Autodesk Inventor part; units mm, degrees
ref_plane "YZ Plane" through (0, 0, 0) normal (1, 0, 0) x (0, 1, 0)
ref_plane "XZ Plane" through (0, 0, 0) normal (0, 1, 0) x (-1, 0, 0)
ref_plane "XY Plane" through (0, 0, 0) normal (0, 0, 1) x (1, 0, 0)
sketch "Sketch1" plane through (0, 0, 0) normal (0, 0, 1) x (1, 0, 0)
  line L0 (-12.4142, 25.4) -> (12.4142, 25.4)
  line L1 (12.4142, 25.4) -> (12.4142, -25.4)
  line L2 (12.4142, -25.4) -> (-12.4142, -25.4)
  line L3 (-12.4142, -25.4) -> (-12.4142, 25.4)
  circle A0 centre (-9.2393, 22.225) radius 2.1844
  circle A1 centre (-9.2393, -22.225) radius 2.1844
  circle A2 centre (9.2393, -22.225) radius 2.1844
  circle A3 centre (9.2393, 22.225) radius 2.1844
  point P0 (0, 0)
  point P1 (-12.4143, 0)
  point P2 (0, 25.4)
  dimension "d0" = 24.8285
  dimension "d1" = 50.8
  dimension "d2" = 4.3688
  dimension "d3" = 47.625
  dimension "d4" = 3.175
  dimension "d5" = 4.3688
  dimension "d6" = 4.3688
  dimension "d7" = 4.3688
  dimension "d8" = 3.175
  dimension "d9" = 3.175
extrude "Extrusion1" add sketch "Sketch1" against normal blind 9.398
properties part number "Ch7(5) Part 9 Cover Plate"
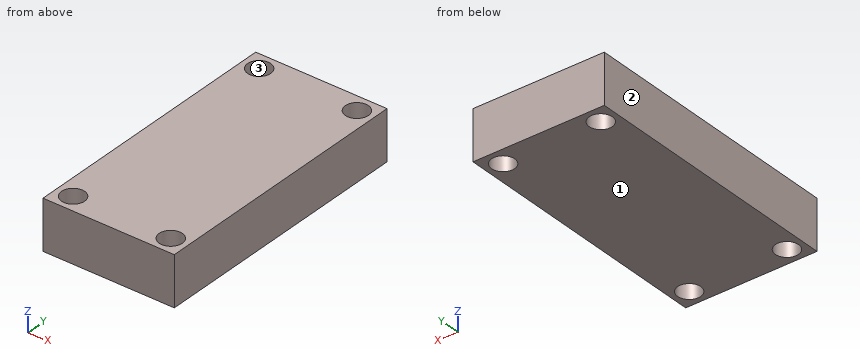
Geometry: final body of the model. Coordinates: model frame, mm. Face numbers are marked on the shaded views. Give positions to 0.01 mm unless a question says otherwise; leave off trailing zeros. Write each loop counter-clockwise with the first axis right and the second up, starting at its lowest first coordinate (ties: lowest second). Pieces come first, ordered by that corner, then holes. Notation, with made-up numbers: M -34,-6 L 23,-6 A5 cw 23,2 Z; hole C -20,33 d4. An arc over 180 degrees is marked long. Answer in a Markdown table with one row per item. Add a question column.
(1) Ray query, line 1 (Y direction, x = -9.25, z = -2); line 2 (Y direction, x = 11, z = -2.5); line 3 (X direction, y = 23.5, z = -8). Return the intervals inside material, ascending.
(2) Section A-A on z = -5.5. Return loops of the section in (x, y) (3 decimals).
(3) Mould query, pull axis X, two halves, no side actions, for the marked faces 1, 2 and 3. Classes: +X half, -X half, draft (parallel to the pull), parting line (faces both ways), or undercut.
(4) Section B-B on x = 9. Return loops of the section in (y, z), and give its area (3 significant figures).
Result set:
| question | item | result |
|---|---|---|
| 1 | line 1 | y = -25.4 to -24.41, -20.04 to 20.04, 24.41 to 25.4 |
| 1 | line 2 | y = -25.4 to -23.52, -20.93 to 20.93, 23.52 to 25.4 |
| 1 | line 3 | x = -12.41 to -11.01, -7.47 to 7.47, 11.01 to 12.41 |
| 2 | outline | M -12.414,-25.4 L 12.414,-25.4 L 12.414,25.4 L -12.414,25.4 Z; hole C -9.239,-22.225 d4.369; hole C -9.239,22.225 d4.369; hole C 9.239,-22.225 d4.369; hole C 9.239,22.225 d4.369 |
| 3 | face 1 | draft |
| 3 | face 2 | -X half |
| 3 | face 3 | undercut |
| 4 | outline | M -25.4,-9.4 L -24.4,-9.4 L -24.4,0 L -25.4,0 Z; M -20.05,-9.4 L 20.05,-9.4 L 20.05,0 L -20.05,0 Z; M 24.4,-9.4 L 25.4,-9.4 L 25.4,0 L 24.4,0 Z |
| 4 | area | 396 mm^2 |
